Here's how the part is built. I have some questions about the finished solid (model axes, mm). Face numbers are marked on the shaded views. A direction names the side the tool comes from. Coordinates: 2 decimals unless noted, no trailing zeros. Write each loop counter-clockwise with the first axis right and the second up, starting at its lowest first coordinate (ties: lowest second). Pieces come first, ordered by that corner, then holes. Notation, with made-up numbers: (78, 29.5) -> (136, 29.5) arc R30 ccw to (136, 56.5) -> close; hole circle Ø1 at (-19.75, -29). An arc over 180 degrees is marked (long way). Put each result on its own line as item: value.
```python
from build123d import *

# Parameters (mm, degrees)
SKETCH_1_W                    = 80
SKETCH_1_H                    = 35
EXTRUDE_1_DEPTH               = 14
SKETCH_2_W                    = 20
SKETCH_2_H                    = 35
EXTRUDE_2_DEPTH               = 26
HOLE_WIZARD_M20_1_D           = 7
HOLE_WIZARD_M20_1_CBORE_D     = 12
HOLE_WIZARD_M20_1_CBORE_DEPTH = 8
PATTERN_LINEAR_1_COUNT        = 2
PATTERN_LINEAR_1_PITCH        = 60
PATTERN_LINEAR_1_COUNT_DIR2   = 2
PATTERN_LINEAR_1_PITCH_DIR2   = 15
SKETCH_5_R                    = 2.5
CUT_EXTRUDE_1_DEPTH           = 67.379590237
PATTERN_LINEAR_2_COUNT        = 2
PATTERN_LINEAR_2_PITCH        = 13
PATTERN_LINEAR_2_COUNT_DIR2   = 2
PATTERN_LINEAR_2_PITCH_DIR2   = 15


with BuildPart() as part:
    # 草图1 → 凸台-拉伸1 (new body)
    with BuildSketch(Plane(origin=(0, 0, 0), x_dir=(1, 0, 0), z_dir=(0, 1, 0))):
        Rectangle(SKETCH_1_W, SKETCH_1_H)
    extrude(amount=EXTRUDE_1_DEPTH)

    # 草图2 → 凸台-拉伸2 (add)
    with BuildSketch(Plane(origin=(0, 14, 0), x_dir=(1, 0, 0), z_dir=(0, 1, 0))):
        Rectangle(SKETCH_2_W, SKETCH_2_H)
    extrude(amount=EXTRUDE_2_DEPTH)

    # M20 六角头螺栓的柱形沉头孔1 (through all)
    with Locations(Plane(origin=(0, 14, 0), x_dir=(1, 0, 0), z_dir=(0, 1, 0))):
        with Locations((-30, 7.5)):
            hole_wizard_m20_1 = CounterBoreHole(HOLE_WIZARD_M20_1_D / 2, HOLE_WIZARD_M20_1_CBORE_D / 2, HOLE_WIZARD_M20_1_CBORE_DEPTH)

    # 阵列(线性)1: Hole Wizard M20 _1 2 × 2
    with Locations(*[(i * PATTERN_LINEAR_1_PITCH, 0, j * PATTERN_LINEAR_1_PITCH_DIR2) for i in range(PATTERN_LINEAR_1_COUNT) for j in range(PATTERN_LINEAR_1_COUNT_DIR2) if (i, j) != (0, 0)]):
        add(hole_wizard_m20_1, mode=Mode.SUBTRACT)

    # 草图5 → 切除-拉伸1 (cut, through all)
    with BuildSketch(Plane.ZY.offset(10)):
        with Locations((-7.5, 21)):
            Circle(SKETCH_5_R)
    cut_extrude_1 = extrude(amount=-CUT_EXTRUDE_1_DEPTH, mode=Mode.SUBTRACT)

    # 阵列(线性)2: Cut-Extrude 1 2 × 2
    with Locations(*[(0, j * PATTERN_LINEAR_2_PITCH_DIR2, i * PATTERN_LINEAR_2_PITCH) for i in range(PATTERN_LINEAR_2_COUNT) for j in range(PATTERN_LINEAR_2_COUNT_DIR2) if (i, j) != (0, 0)]):
        add(cut_extrude_1, mode=Mode.SUBTRACT)


solid = part.part
```
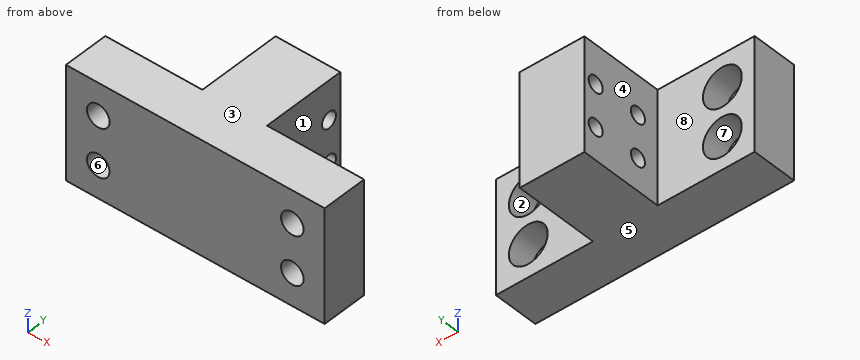
Item 1: Imagine slicing it at B-B on z = -7.5. State how many separate pieces and enclosed holes the cut face has, then the cut area to 3 significant figures.
Output:
separate pieces: 5
enclosed holes: 0
area: 1,160 mm²
Item 2: Imagine slicing it at D-D on x = 2. Write out the boundary of the cut face in (y, z).
Output:
outline: (0, -17.5) -> (40, -17.5) -> (40, 17.5) -> (0, 17.5) -> close; hole circle Ø5 at (21, -7.5); hole circle Ø5 at (21, 5.5); hole circle Ø5 at (36, -7.5); hole circle Ø5 at (36, 5.5)
Item 3: Which directions (+Z, -Z, +X, -X, +Y, -Y) give clear straight access to the entire face, cutting with the end or side of a thin tool? Please do the marked faces 1, 2, 3 and 4.
Output:
face 1: +Z, -Z, +X, +Y
face 2: +Y
face 3: +Z, +X, -X, +Y, -Y
face 4: +Z, -Z, -X, +Y
Item 4: Imagine slicing it at C-C on x = 30. Write out the boundary of the cut face in (y, z).
Output:
outline: (0, -17.5) -> (14, -17.5) -> (14, -13.5) -> (6, -13.5) -> (6, -11) -> (0, -11) -> close; (0, -4) -> (6, -4) -> (6, -1.5) -> (14, -1.5) -> (14, 1.5) -> (6, 1.5) -> (6, 4) -> (0, 4) -> close; (0, 11) -> (6, 11) -> (6, 13.5) -> (14, 13.5) -> (14, 17.5) -> (0, 17.5) -> close
Item 5: For P1, Ø15.5, axis at x = 30, z = -7.5, coming from the -Y side; P2, Ø3, axis at y = 20, z = 10, coming from the +X side; P3, Ø2, axis at x = 21.5, z = 12, coming from the +Y side; P4, Ø11, axis at x = 30, z = 7.5, coming from the +Y side, each with a flat end and sliding along its axis, tell me the tip position at first contact or that it passes through.
Output:
P1: stops at y = 0
P2: stops at x = 10
P3: stops at y = 14
P4: stops at y = 6
Item 6: Please list where these lines run through material, in increasing order: line 1 along Z through (x, y) = (-30, 10); line 2 along X through (y, z) = (9, 7); line 3 along X through (y, z) = (8, 4). Write a range as from..to.
Output:
line 1: z = -17.5..-13.5, -1.5..1.5, 13.5..17.5
line 2: x = -40..-35.98, -24.02..24.02, 35.98..40
line 3: x = -40..-34.87, -25.13..25.13, 34.87..40
Item 7: If we mould it in two halves opening along Z, with no side actions, what happens to the marked faces 5, 6, 7 and 8? For each: released by +Z, released by -Z, zero draft, split by the parting line, or undercut.
Output:
face 5: released by -Z
face 6: undercut
face 7: undercut
face 8: zero draft
Item 8: Imagine slicing it at A-A on y = 36. Write out the boundary of the cut face in (x, z), then the cut area to 3 significant figures.
Output:
outline: (-10, -17.5) -> (10, -17.5) -> (10, -10) -> (-10, -10) -> close; (-10, -5) -> (10, -5) -> (10, 3) -> (-10, 3) -> close; (-10, 8) -> (10, 8) -> (10, 17.5) -> (-10, 17.5) -> close
area: 500 mm²
